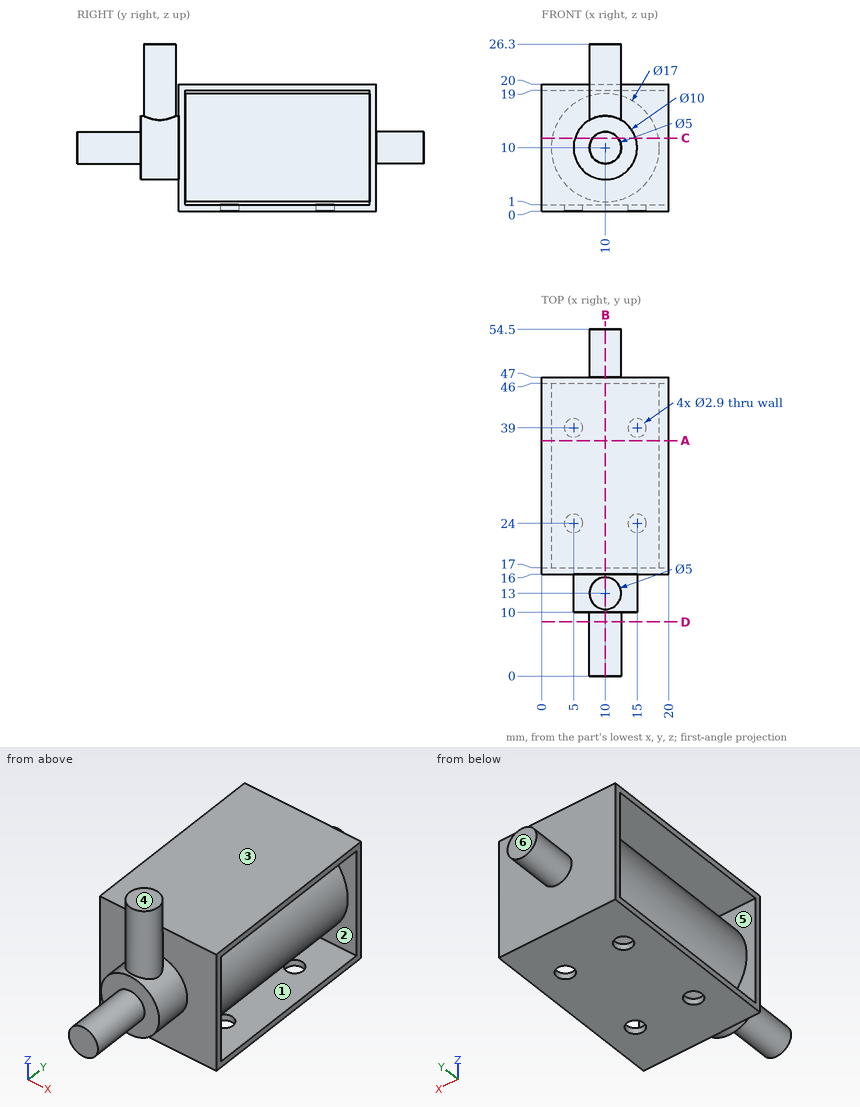
Drawing for the job (mm, zero at the part's lowest x, y, z). A direction names the side the tool comes from. Give positions to 0.01 mm unless a question says otherwise; leave off trailing zeros. Loops run counter-clockwise (first coordinate to the right, second up) from the corner with the lowest first, then second, coordinate; pieces in that order, holes last. Notation, with made-up numbers: M -22,-38.75 L -3,-38.75 A15 cw -3,-10.75 Z; hole C 79,88 d5. An arc over 180 degrees is marked long. Use one line per item in the form item = value.
Item 1: Two-plate mould, pull along Z, no slides. Class the marked faces 4, 5 and 6: pulls with the +Z half, pulls with the -Z half, needs draft (parallel to the pull), parting line crosses it, or undercut.
Determined:
face_4 = pulls with the +Z half
face_5 = undercut
face_6 = needs draft
Item 2: Flat gauge pins, fed straight in: pin 1 (5 mm diameter, centred on x = 12, z = 9.5, fed in from -Y); pin 2 (8 mm diameter, centred on y = 40, z = 5.5, fed in from -X); pin 3 (2 mm diameter, centred on x = 9, y = 26.5, fed in from +Z); pin 4 (2.5 mm diameter, centred on x = 15, y = 24, fed in from -Z). Where does each tip first touch, or does it go through?
Determined:
pin_1 = 0
pin_2 = 1.51
pin_3 = 20
pin_4 = 2.37
Item 3: Drill centre lines: probe 1 along Y at (x, z) = (5, 0.55); probe 2 along X at (y, z) = (24, 0.85); probe 3 along Z at (x, y) = (15.75, 31.5). Where is each one in solid material? Low to high. Write a range as from..to.
Determined:
probe_1 = 16..22.55, 25.45..37.55, 40.45..47
probe_2 = 0..3.55, 6.45..13.55, 16.45..20
probe_3 = 0..1, 3.74..16.26, 19..20
Item 4: Slice it at D-D (y = 8.5). List the corners of the cut face in (x, z).
Determined:
outline = C 10,10 d5
Item 5: Slice it at B-B (x = 10). List the corners of the cut face in (y, z), plus the area to 3 significant figures.
Determined:
outline = M 0,7.5 L 10,7.5 L 10,5 L 16,5 L 16,0 L 47,0 L 47,7.5 L 54.5,7.5 L 54.5,12.5 L 47,12.5 L 47,20 L 16,20 L 16,15 L 15.5,15 L 15.5,26.3 L 10.5,26.3 L 10.5,15 L 10,15 L 10,12.5 L 0,12.5 Z; hole M 17,1 L 46,1 L 46,1.5 L 17,1.5 Z; hole M 17,18.5 L 46,18.5 L 46,19 L 17,19 Z
area = 795 mm2
Item 6: Which spindle directions (+Z, -Z, +X, -X, +Y, -Y) get a long thin tool onto all of the face, cutting with end or side? Do the marked faces 1, 2 and 3. Say none if no direction does.
Determined:
face_1 = +X, -X
face_2 = none
face_3 = +Z, +X, -X, +Y
Item 7: Slice it at C-C (z = 11.5). List the corners of the cut face in (x, y), plus the area to 4 significant figures.
Determined:
outline = M 0,16 L 5.23,16 L 5.23,10 L 8,10 L 8,0 L 12,0 L 12,10 L 14.77,10 L 14.77,16 L 20,16 L 20,17 L 18.37,17 L 18.37,46 L 20,46 L 20,47 L 12,47 L 12,54.5 L 8,54.5 L 8,47 L 0,47 L 0,46 L 1.63,46 L 1.63,17 L 0,17 Z
area = 652.5 mm2
Item 8: Slice it at A-A (y = 37). List the corners of the cut face in (x, z), plus the area to 3 significant figures.
Determined:
outline = M 0,0 L 20,0 L 20,1 L 0,1 Z; M 0,19 L 20,19 L 20,20 L 0,20 Z; C 10,10 d17
area = 267 mm2
